Could you check a few things on this model? Use its own coordinates, in mm. A direction names the side the tool comes from. Round coordinates to 2 decimals unless told otherwise and drop trailing zeros. Loops run counter-clockwise (first coordinate to the right, second up) from the corner with the lowest first, then second, coordinate; pieces in that order, holes last. Notation, with made-up numbers: (43.25, 86) -> (72.25, 86) arc R29 cw to (72.25, 117) -> close; hole circle Ø7 at (20, 12.25). An arc over 180 degrees is marked (long way). Put each result on its own line as item: value. Start each with the question number.
1. Imagine slicing it at D-D, the plane z = 0.6. Please give me the cut outline in (x, y).
2. If we mould it in two halves opening along Y, with no side actions, what happens to faces 3 (the flat face through (34, 1, 2)), 4 (the cylindrical face through (-1.951, 71.286, 0.986)), 5 (the cylindrical face through (-17.34, 78.1, 0.99))? For each: pulls with the +Y half, pulls with the -Y half, needs draft (parallel to the pull), parting line crosses it, or undercut.
3. Imagine slicing it at C-C, the plane x = -20. Please give me the cut outline in (y, z), and give its area (3 significant figures).
4. Imagine slicing it at A-A, the plane x = 0. Please give me the cut outline in (y, z).
5. Which directions (+Z, -Z, +X, -X, +Y, -Y) give clear straight access to the entire face, cutting with the end or side of a thin tool? Please do faces 1 (the flat face through (34, 1, 0)), 2 (the flat face through (-20.98, 20.74, 0.99)).
6. I'm going to push flat-ended pins straight in: P1, Ø0.6, axis at y = -3, z = 0.5, coming from the +X side; P2, Ø14.5, axis at x = 0, y = -62.5, coming from the +Z side. Where does each tip first touch, or does it pass through?
7. I need wall thicknesses on line 1 (Y direction, x = 0, z = 1.2); line 2 (X direction, y = -2.5, z = 1); line 3 (Y direction, x = 62.5, z = 1.3). Which ranges of each line are inside material? Lowest first, please. Write a range as [from, to].
Autodesk Inventor part; units mm, degrees
ref_plane "YZ Plane" through (0, 0, 0) normal (1, 0, 0) x (0, 1, 0)
ref_plane "XZ Plane" through (0, 0, 0) normal (0, 1, 0) x (-1, 0, 0)
ref_plane "XY Plane" through (0, 0, 0) normal (0, 0, 1) x (1, 0, 0)
sketch "Sketch1" plane through (0, 0, 0) normal (0, 0, 1) x (1, 0, 0)
  circle A0 centre (0, 0) radius 62.5 construction
  circle A1 centre (0, 0) radius 29.5 construction
  circle A2 centre (0, 0) radius 80
  line L0 (12.2193, 29.5) -> (29.5, 12.2193)
  line L1 (29.5, 12.2193) -> (29.5, -12.2193)
  line L2 (29.5, -12.2193) -> (12.2193, -29.5)
  line L3 (12.2193, -29.5) -> (-12.2193, -29.5)
  line L4 (-12.2193, -29.5) -> (-29.5, -12.2193)
  line L5 (-29.5, -12.2193) -> (-29.5, 12.2193)
  line L6 (-29.5, 12.2193) -> (-12.2193, 29.5)
  line L7 (-12.2193, 29.5) -> (12.2193, 29.5)
  circle A3 centre (0, 62.5) radius 9
  circle A4 centre (-62.5, 0) radius 9
  circle A5 centre (0, -62.5) radius 9
  circle A6 centre (62.5, 0) radius 9
  point P0 (0, 29.5)
  dimension "D_b_c" = 125
  dimension "D_min" = 59
  dimension "D_max" = 160
  dimension "Blt_hl" = 18
  dimension "d177" = 360
extrude "Plate5" add sketch "Sketch1" along normal blind 2
properties part number "PRS 1200-82 funnel FLANGE" material "Stainless Steel"
Entries:
1. outline: circle Ø160 at (0, 0); hole circle Ø18 at (-62.5, 0); hole (-29.5, -12.22) -> (-12.22, -29.5) -> (12.22, -29.5) -> (29.5, -12.22) -> (29.5, 12.22) -> (12.22, 29.5) -> (-12.22, 29.5) -> (-29.5, 12.22) -> close; hole circle Ø18 at (0, -62.5); hole circle Ø18 at (0, 62.5); hole circle Ø18 at (62.5, 0)
2. face 3: needs draft
2. face 4: undercut
2. face 5: parting line crosses it
3. outline: (-77.46, 0) -> (-21.72, 0) -> (-21.72, 2) -> (-77.46, 2) -> close; (21.72, 0) -> (77.46, 0) -> (77.46, 2) -> (21.72, 2) -> close
3. area: 223 mm^2
4. outline: (-80, 0) -> (-71.5, 0) -> (-71.5, 2) -> (-80, 2) -> close; (-53.5, 0) -> (-29.5, 0) -> (-29.5, 2) -> (-53.5, 2) -> close; (29.5, 0) -> (53.5, 0) -> (53.5, 2) -> (29.5, 2) -> close; (71.5, 0) -> (80, 0) -> (80, 2) -> (71.5, 2) -> close
5. face 1: -Z, +X, -X, +Y, -Y
5. face 2: +Z, -Z
6. P1: x = 79.95
6. P2: through
7. line 1: [-80, -71.5], [-53.5, -29.5], [29.5, 53.5], [71.5, 80]
7. line 2: [-79.96, -71.15], [-53.85, -29.5], [29.5, 53.85], [71.15, 79.96]
7. line 3: [-49.94, -9], [9, 49.94]
